Input: part model. Units: mm. Frame: model coordinates. Face numbers are marked on the shaded views. Coordinates: 2 decimals unless noted, no trailing zeros. Order: outer loops, then holes, each group sorted by start corner. A loop starts at its lowest first (then second) coordinate and runs counter-clockwise, first axis right, second up. Notation, with made-up numbers: M 63.5,-13 L 112.5,-13 A23 cw 112.5,11 Z; hole C -18,10 d5. An arc over 180 degrees is marked long. Answer in a Markdown table with one row per item.
from build123d import *

# Parameters (mm, degrees)
EXTRUDE_1_DEPTH = 6.4
SKETCH_2_R      = 5
EXTRUDE_2_DEPTH = 30
CHAMFER_1_SIZE  = 0.828


with BuildPart() as part:
    # Эскиз1 → Бобышка-Вытянуть1 (new body)
    with BuildSketch(Plane.XY):
        Polygon((-4.907477288, 8.5), (-9.814954576, 0), (-4.907477288, -8.5), (4.907477288, -8.5), (9.814954576, 0), (4.907477288, 8.5), align=None)
    extrude(amount=EXTRUDE_1_DEPTH)

    # Эскиз2 → Бобышка-Вытянуть2 (add)
    with BuildSketch(Plane.XY.offset(6.4)):
        Circle(SKETCH_2_R)
    extrude(amount=EXTRUDE_2_DEPTH)

    # Эскиз3 → Вырез-Повернуть1 (revolve, cut)
    with BuildSketch(Plane(origin=(0, 0, 0), x_dir=(0, 0, -1), z_dir=(1, 0, 0))):
        Polygon((0, 8.5), (0, 11.5), (-1.732050808, 11.5), align=None)
    revolve(axis=Axis((0, 0, 1000), (0, 0, -1)), mode=Mode.SUBTRACT)

    # Фаска1
    chamfer_1_edges = [part.edges().sort_by_distance(p)[0] for p in [
        (-5, 0, 36.4),
    ]]
    chamfer(chamfer_1_edges, length=CHAMFER_1_SIZE)


solid = part.part
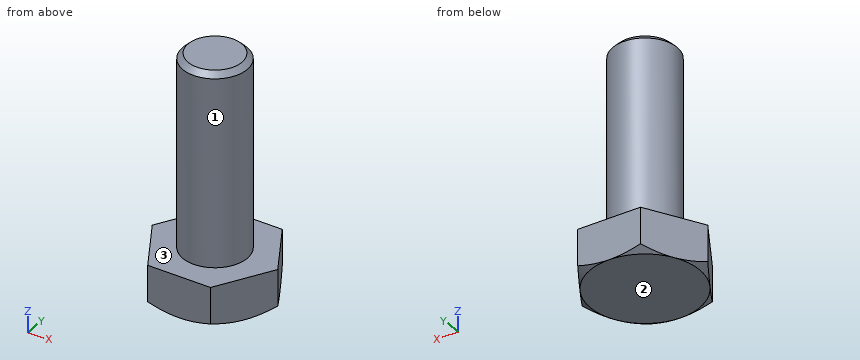
1) Cut plane A-A, the plane z = 10. Output: boundary loops of the cut face in (x, y), and give its area (3 significant figures).
Resolved:
| item | result |
|---|---|
| outline | C 0,0 d10 |
| area | 78.5 mm2 |
2) Mould query, pull axis Z, two halves, no side actions, for the marked faces 1, 2 and 3. Classes: +Z half, -Z half, draft (parallel to the pull), parting line (faces both ways), or undercut.
Resolved:
| item | result |
|---|---|
| face 1 | draft |
| face 2 | -Z half |
| face 3 | +Z half |
3) Material intervals for probe 1 along Z at (x, y) = (-0.75, -6); probe 2 along Y at (x, z) = (1, 16); probe 3 along Z at (x, y) = (-0.25, -4.75), sorted ascending.
Resolved:
| item | result |
|---|---|
| probe 1 | z = 0 to 6.4 |
| probe 2 | y = -4.9 to 4.9 |
| probe 3 | z = 0 to 35.82 |
4) Contact query for flat-ended pins moving along their axis: pin 1 (4 mm diameter, centred on x = -4, z = 23.5, fed in from +Y); pin 2 (4 mm diameter, centred on y = -3.5, z = 31.5, fed in from -X); pin 3 (2 mm diameter, centred on x = 0, z = 20, fed in from -Y). Output: stop coordinate, or through.
Resolved:
| item | result |
|---|---|
| pin 1 | stops at y = 4.58 |
| pin 2 | stops at x = -4.77 |
| pin 3 | stops at y = -5 |
